```python
from build123d import *

# Parameters (mm, degrees)
F0_R     = 23.8125
F1_DEPTH = 2.667


with BuildPart() as f1:
    # F0 (on Front) → F1 (new body)
    with BuildSketch(Plane.XZ):
        with BuildLine():
            ThreePointArc((-65.964614, 2.051073), (-65.869192, 3.084735), (-65.735439, 4.114139))
            Line((-65.735439, 4.114139), (-68.707, 4.114139))
            Line((-68.707, 4.114139), (-68.707, 2.051073))
            Line((-68.707, 2.051073), (-65.964614, 2.051073))
        make_face()
        with BuildLine():
            ThreePointArc((-65.735439, -4.114139), (-36.037302, -27.863756), (-10.16, 0))
            ThreePointArc((-10.16, 0), (-10.160749, 0.204565), (-10.162995, 0.40912))
            ThreePointArc((-10.162995, 0.40912), (-10.266731, 2.439818), (-10.517878, 4.457595))
            ThreePointArc((-10.517878, 4.457595), (-38.273785, 27.93946), (-65.735439, 4.114139))
            ThreePointArc((-65.735439, 4.114139), (-65.869192, 3.084735), (-65.964614, 2.051073))
            ThreePointArc((-65.964614, 2.051073), (-66.04, 0), (-65.964614, -2.051073))
            ThreePointArc((-65.964614, -2.051073), (-65.869192, -3.084735), (-65.735439, -4.114139))
        make_face()
        with Locations((-38.1, 0)):
            Circle(F0_R, mode=Mode.SUBTRACT)
        with BuildLine():
            Line((-68.707, -4.114139), (-65.735439, -4.114139))
            ThreePointArc((-65.735439, -4.114139), (-65.869192, -3.084735), (-65.964614, -2.051073))
            Line((-65.964614, -2.051073), (-68.707, -2.051073))
            Line((-68.707, -2.051073), (-68.707, -4.114139))
        make_face()
        with BuildLine():
            ThreePointArc((-10.517878, 4.457595), (-10.266731, 2.439818), (-10.162995, 0.40912))
            ThreePointArc((-10.162995, 0.40912), (0, 3.600017), (10.162995, 0.40912))
            ThreePointArc((10.162995, 0.40912), (10.266731, 2.439818), (10.517878, 4.457595))
            ThreePointArc((10.517878, 4.457595), (0, 7.902232), (-10.517878, 4.457595))
        make_face()
        with BuildLine():
            ThreePointArc((10.517878, 4.457595), (10.266731, 2.439818), (10.162995, 0.40912))
            ThreePointArc((10.162995, 0.40912), (35.83335, -27.847907), (65.735439, -4.114139))
            ThreePointArc((65.735439, -4.114139), (65.869192, -3.084735), (65.964614, -2.051073))
            ThreePointArc((65.964614, -2.051073), (66.021147, -1.026229), (66.04, 0))
            ThreePointArc((66.04, 0), (66.021147, 1.026229), (65.964614, 2.051073))
            ThreePointArc((65.964614, 2.051073), (65.869192, 3.084735), (65.735439, 4.114139))
            ThreePointArc((65.735439, 4.114139), (38.273785, 27.93946), (10.517878, 4.457595))
        make_face()
        with Locations((38.1, 0)):
            Circle(F0_R, mode=Mode.SUBTRACT)
        with BuildLine():
            ThreePointArc((65.964614, -2.051073), (65.869192, -3.084735), (65.735439, -4.114139))
            Line((65.735439, -4.114139), (68.707, -4.114139))
            Line((68.707, -4.114139), (68.707, -2.051073))
            Line((68.707, -2.051073), (65.964614, -2.051073))
        make_face()
        with BuildLine():
            Line((68.707, 4.114139), (65.735439, 4.114139))
            ThreePointArc((65.735439, 4.114139), (65.869192, 3.084735), (65.964614, 2.051073))
            Line((65.964614, 2.051073), (68.707, 2.051073))
            Line((68.707, 2.051073), (68.707, 4.114139))
        make_face()
    extrude(amount=F1_DEPTH)


solid = f1.part
```
Geometry check sheet. Reference: the model listing, model coordinates, mm. A direction names the side the tool comes from. Coordinates: 2 decimals unless noted, no trailing zeros. Order: outer loops, then holes, each group sorted by start corner. A loop starts at its lowest first (then second) coordinate and runs counter-clockwise, first axis right, second up. Notation, with made-up numbers: M 51,72 L 73,72 A9 cw 73,80 Z; hole C -36.5,68 d8. An arc over 180 degrees is marked long. One line per question, with ' | ' between items. Start each with the question number.
Item 1: Cross-section at D-D on x = -21. Enter the section's corners in (y, z), then the cut area to 3 significant figures.
Item 2: Set-up check for faces 4 (the flat face through (67, -1, -4.114)), 5 (the flat face through (-67, -1, 4.114)), 6 (the flat face through (67, -1, 4.114)), 7 (the flat face through (67, -1, -2.051)): record each of +Z, -Z, +X, -X, +Y, -Y from which the full face is reachable in a straight line by a thin tool's end or side.
Item 3: Draft check along Z on faces 1 (the cylindrical face through (-0.2, -1.3, 3.6)), 2 (the flat face through (5, -2.667, 4)), 3 (the cylindrical face through (-66.04, -1.31, 0.03)). Enter one of: pulls with the +Z half, pulls with the -Z half, needs draft (parallel to the pull), parting line crosses it, or undercut.
Item 4: Cross-section at C-C on z = -19.5. Enter the section's corners in (x, y), then the cut area to 3 significant figures.
Item 5: Cross-section at A-A on y = -1. Enter the section's corners in (x, z) (1 decimal), then the cut area to 3 significant figures.
Item 6: Gauge pin test, flat ends, axial feed: pin 1 (0.8 mm diameter, centred on x = 67, y = -1.5, fed in from -Z); pin 2 (1.3 mm diameter, centred on x = 68, y = -1.5, fed in from +Z); pin 3 (1 mm diameter, centred on y = -0.5, z = 15.5, fed in from -X). Record the tip position at first contact, or that the pin passes through.
Item 7: Cross-section at B-B on x = -38.1. Enter the section's corners in (y, z).
Item 8: Material ranges on L1, parallel to X at y = -0.2, z = -13; L2, parallel to Z at x = 38, y = -2.4; L3, parallel to X at y = -1.15, z = -12, recorded low to high. Write a range as [from, to].
Findings:
1) outline: M -2.67,-22.1 L 0,-22.1 L 0,-16.57 L -2.67,-16.57 Z; M -2.67,16.57 L 0,16.57 L 0,22.1 L -2.67,22.1 Z | area: 29.5 mm²
2) face 4: -Z, +X, +Y, -Y | face 5: +Z, -X, +Y, -Y | face 6: +Z, +X, +Y, -Y | face 7: +X, +Y, -Y
3) face 1: pulls with the -Z half | face 2: needs draft | face 3: undercut
4) outline: M -58.11,-2.67 L -51.77,-2.67 L -51.77,0 L -58.11,0 Z; M -24.43,-2.67 L -18.09,-2.67 L -18.09,0 L -24.43,0 Z; M 18.09,-2.67 L 24.43,-2.67 L 24.43,0 L 18.09,0 Z; M 51.77,-2.67 L 58.11,-2.67 L 58.11,0 L 51.77,0 Z | area: 67.7 mm²
5) outline: M -68.7,-4.1 L -65.7,-4.1 A27.9 ccw -10.2,0 A28 ccw -10.2,0.4 A17.8 cw 10.2,0.4 A27.9 ccw 65.7,-4.1 L 68.7,-4.1 L 68.7,-2.1 L 66,-2.1 A27.9 ccw 66,0 A27.9 ccw 66,2.1 L 68.7,2.1 L 68.7,4.1 L 65.7,4.1 A27.9 ccw 10.5,4.5 A17.8 ccw -10.5,4.5 A27.9 ccw -65.7,4.1 L -68.7,4.1 L -68.7,2.1 L -66,2.1 A27.9 ccw -66,-2.1 L -68.7,-2.1 Z; hole C -38.1,0 d47.6; hole C 38.1,0 d47.6 | area: 1,450 mm²
6) pin 1: stops at z = -4.11 | pin 2: stops at z = 4.11 | pin 3: stops at x = -61.67
7) outline: M -2.67,-27.94 L 0,-27.94 L 0,-23.81 L -2.67,-23.81 Z; M -2.67,23.81 L 0,23.81 L 0,27.94 L -2.67,27.94 Z
8) L1: x = [-62.83, -58.05], [-18.15, -13.37], [13.37, 18.15], [58.05, 62.83] | L2: z = [-27.94, -23.81], [23.81, 27.94] | L3: x = [-63.33, -58.67], [-17.53, -12.87], [12.87, 17.53], [58.67, 63.33]
